Design review of the part shown in the three views and the two pictorial views. Dimensions are in mm from the part's minimum x, y and z. A direction names the side the tool comes from. Give positions to 0.01 mm unless a question says otherwise; leave off trailing zeros. Order: outer loops, then holes, each group sorted by start corner. A loop starts at its lowest first (then second) coordinate and runs counter-clockwise, first axis right, second up.
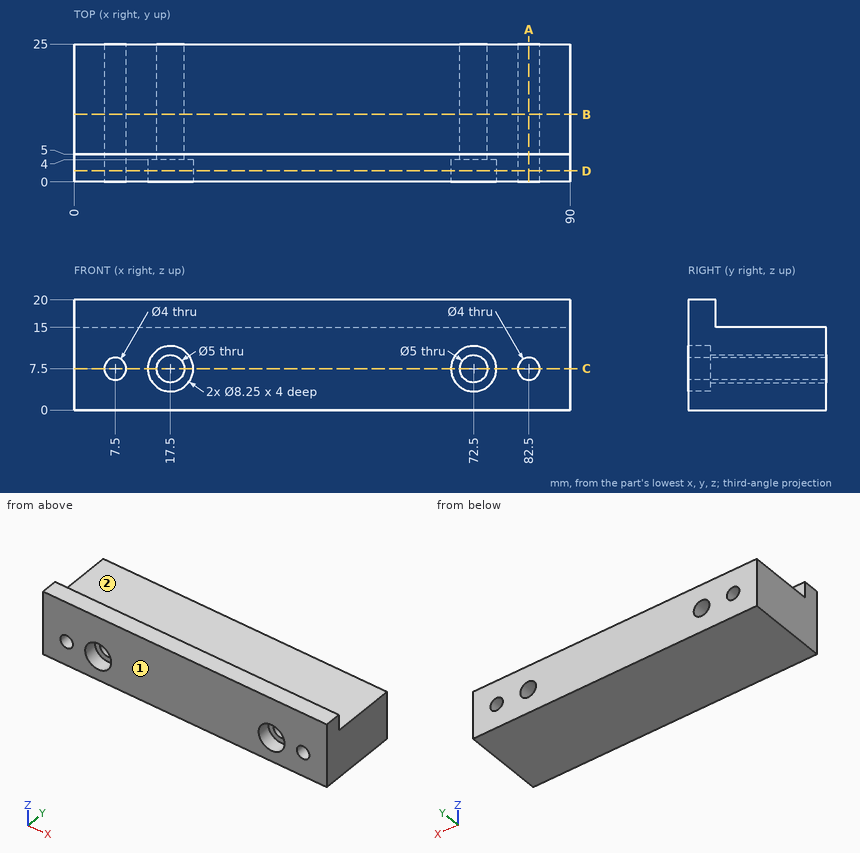
1) To check wall thickness, follow line 1 (Z direction, x = 72.5, y = 15); line 2 (X direction, y = 22.25, z = 9); line 3 (X direction, y = 5.5, z = 7). State the ranges of each line that lie inside material, in increasing order.
Answer sheet:
line 1: z = 0 to 5, 10 to 15
line 2: x = 0 to 6.18, 8.82 to 15.5, 19.5 to 70.5, 74.5 to 81.18, 83.82 to 90
line 3: x = 0 to 5.56, 9.44 to 15.05, 19.95 to 70.05, 74.95 to 80.56, 84.44 to 90
2) We need section C-C on z = 7.5. Give the boundary of the cut face in (x, y) (3 decimals), then the cut area to 3 significant figures.
Answer sheet:
outline: (0, 0) - (5.5, 0) - (5.5, 25) - (0, 25) - close; (9.5, 0) - (13.375, 0) - (13.375, 4) - (15, 4) - (15, 25) - (9.5, 25) - close; (20, 4) - (21.625, 4) - (21.625, 0) - (68.375, 0) - (68.375, 4) - (70, 4) - (70, 25) - (20, 25) - close; (75, 4) - (76.625, 4) - (76.625, 0) - (80.5, 0) - (80.5, 25) - (75, 25) - close; (84.5, 0) - (90, 0) - (90, 25) - (84.5, 25) - close
area: 1,770 mm2
3) We need section B-B on y = 12.25. Give the boundary of the cut face in (x, z), then the cut area to 3 significant figures.
Answer sheet:
outline: (0, 0) - (90, 0) - (90, 15) - (0, 15) - close; hole circle Ø4 at (7.5, 7.5); hole circle Ø5 at (17.5, 7.5); hole circle Ø5 at (72.5, 7.5); hole circle Ø4 at (82.5, 7.5)
area: 1,290 mm2
4) We need section D-D on y = 2. Give the boundary of the cut face in (x, z) (3 decimals), then the cut area to 3 significant figures.
Answer sheet:
outline: (0, 0) - (90, 0) - (90, 20) - (0, 20) - close; hole circle Ø4 at (7.5, 7.5); hole circle Ø8.25 at (17.5, 7.5); hole circle Ø8.25 at (72.5, 7.5); hole circle Ø4 at (82.5, 7.5)
area: 1,670 mm2
5) We need section A-A on x = 82.5. Give the boundary of the cut face in (y, z).
Answer sheet:
outline: (0, 0) - (25, 0) - (25, 5.5) - (0, 5.5) - close; (0, 9.5) - (25, 9.5) - (25, 15) - (5, 15) - (5, 20) - (0, 20) - close
6) Clearance check with flat-ended pins moving along their axes: pin 1 (8 mm diameter, centred on x = 77.5, y = 12.5, fed in from +Z); pin 2 (10.5 mm diameter, centred on x = 72.5, z = 7.5, fed in from +Y); pin 3 (2.5 mm diameter, centred on x = 71, z = 5.5, fed in from -Y). State where each tip first meets the part, or that it passes through.
Answer sheet:
pin 1: stops at z = 15
pin 2: stops at y = 25
pin 3: stops at y = 4
7) Tool access review of the marked faces 1 and 2: name each direction out of +Z, -Z, +X, -X, +Y, -Y from which nothing blocks a thin tool from reaching the whole face with its end or side.
Answer sheet:
face 1: +Z, -Z, +X, -X, -Y
face 2: +Z, +X, -X, +Y
